```python
from build123d import *

# Parameters (mm, degrees)
F0_W           = 131.6228
F0_H           = 90.3224
F1_DEPTH       = 3
F2_W           = 131.6228
F2_H           = 90.3224
F2_W_2         = 123.6228
F2_H_2         = 82.3224
F3_DEPTH       = 25
F4_W           = 123.6228
F4_H           = 4
F5_DEPTH       = 25
F6_R           = 2.5
F7_W           = 10
F7_H           = 4
F8_DEPTH       = 5
F10_DEPTH      = 25
F10_DEPTH_BACK = 95.8124
F12_D          = 2.5
F12_DEPTH      = 1
F12_TIP        = 0.7510757738
F14_D          = 2.5
F14_DEPTH      = 1
F14_TIP        = 0.7510757738
F16_D          = 2.5
F16_DEPTH      = 1
F16_TIP        = 0.7510757738
F18_D          = 2.5
F18_DEPTH      = 1
F18_TIP        = 0.7510757738
F19_W          = 123.6228
F19_H          = 82.3224
F20_DEPTH      = 3


with BuildPart() as f1:
    # F0 (on Top) → F1 (new body)
    with BuildSketch(Plane.XY):
        Rectangle(F0_W, F0_H)
    extrude(amount=F1_DEPTH)

    # F2 (on face) → F3 (join)
    with BuildSketch(Plane.XY.offset(3)):
        Rectangle(F2_W, F2_H)
        Rectangle(F2_W_2, F2_H_2, mode=Mode.SUBTRACT)
    extrude(amount=F3_DEPTH)

    # F4 (on face) → F5 (join)
    with BuildSketch(Plane.XY.offset(3)):
        Rectangle(F4_W, F4_H)
    extrude(amount=F5_DEPTH)

    # F6
    f6_edges = [f1.edges().sort_by_distance(p)[0] for p in [
        (65.8114, 45.1612, 14),
        (65.8114, -45.1612, 14),
        (-65.8114, -45.1612, 14),
        (-65.8114, 45.1612, 14),
        (0, 45.1612, 0),
        (-65.8114, 0, 0),
        (0, -45.1612, 0),
        (65.8114, 0, 0),
    ]]
    fillet(f6_edges, radius=F6_R)

    # F7 (on face) → F8 (join)
    with BuildSketch(Plane(origin=(0, 45.1612, 0), x_dir=(-1, 0, 0), z_dir=(0, 1, 0))):
        with Locations((-35, 26)):
            Rectangle(F7_W, F7_H)
        with Locations((35, 26)):
            Rectangle(F7_W, F7_H)
    extrude(amount=F8_DEPTH)

    # F9 (on face) → F10 (cut, two sides)
    with BuildSketch(Plane(origin=(30, 0, 0), x_dir=(0, -1, 0), z_dir=(-1, 0, 0))) as f10_sk:
        with BuildLine():
            ThreePointArc((-50.1612, 26), (-49.5754135624, 27.4142135624), (-48.1612, 28))
            Line((-48.1612, 28), (-50.1612, 28))
            Line((-50.1612, 28), (-50.1612, 26))
        make_face()
        with BuildLine():
            Line((-50.1612, 24), (-48.1612, 24))
            ThreePointArc((-48.1612, 24), (-49.5754135624, 24.5857864376), (-50.1612, 26))
            Line((-50.1612, 26), (-50.1612, 24))
        make_face()
        with BuildLine():
            Line((-45.1612, 25), (-46.4291491924, 25))
            ThreePointArc((-46.4291491924, 25), (-47.1612, 24.2679491924), (-48.1612, 24))
            Line((-48.1612, 24), (-45.1612, 24))
            Line((-45.1612, 24), (-45.1612, 25))
        make_face()
        with BuildLine():
            ThreePointArc((-48.1612, 28), (-47.1612, 27.7320508076), (-46.4291491924, 27))
            Line((-46.4291491924, 27), (-45.1612, 27))
            Line((-45.1612, 27), (-45.1612, 28))
            Line((-45.1612, 28), (-48.1612, 28))
        make_face()
    extrude(amount=-F10_DEPTH, mode=Mode.SUBTRACT)
    extrude(f10_sk.sketch, amount=F10_DEPTH_BACK, mode=Mode.SUBTRACT)

    # F12 (one way)
    with BuildSketch(Plane(origin=(30, 0, 0), x_dir=(0, -1, 0), z_dir=(-1, 0, 0))):
        with Locations((-48.1612, 26)):
            Circle(F12_D / 2)
    extrude(amount=-F12_DEPTH, mode=Mode.SUBTRACT)
    with Locations(Plane(origin=(30, 0, 0), x_dir=(0, -1, 0), z_dir=(-1, 0, 0))):
        with Locations((-48.1612, 26)):
            with Locations((0, 0, -(F12_DEPTH + F12_TIP / 2))):  # 118° drill point
                Cone(0, F12_D / 2, F12_TIP, mode=Mode.SUBTRACT)

    # F14
    with Locations(Plane.YZ.offset(40)):
        with Locations((48.1612, 26)):
            Hole(F14_D / 2, depth=F14_DEPTH)
            with Locations((0, 0, -(F14_DEPTH + F14_TIP / 2))):  # 118° drill point
                Cone(0, F14_D / 2, F14_TIP, mode=Mode.SUBTRACT)

    # F16 (one way)
    with BuildSketch(Plane.YZ.offset(-30)):
        with Locations((48.1612, 26)):
            Circle(F16_D / 2)
    extrude(amount=-F16_DEPTH, mode=Mode.SUBTRACT)
    with Locations(Plane.YZ.offset(-30)):
        with Locations((48.1612, 26)):
            with Locations((0, 0, -(F16_DEPTH + F16_TIP / 2))):  # 118° drill point
                Cone(0, F16_D / 2, F16_TIP, mode=Mode.SUBTRACT)

    # F18
    with Locations(Plane(origin=(-40, 0, 0), x_dir=(0, -1, 0), z_dir=(-1, 0, 0))):
        with Locations((-48.1612, 26)):
            Hole(F18_D / 2, depth=F18_DEPTH)
            with Locations((0, 0, -(F18_DEPTH + F18_TIP / 2))):  # 118° drill point
                Cone(0, F18_D / 2, F18_TIP, mode=Mode.SUBTRACT)

    # F19 (on face) → F20 (cut)
    with BuildSketch(Plane.XY.offset(28)):
        Rectangle(F19_W, F19_H)
    extrude(amount=-F20_DEPTH, mode=Mode.SUBTRACT)


solid = f1.part
```
Read the model definition and answer for the solid it produces. Units are mm, in the model's axes. A direction names the side the tool comes from. Coordinates: 2 decimals unless noted, no trailing zeros. Write each loop counter-clockwise with the first axis right and the second up, starting at its lowest first coordinate (ties: lowest second). Pieces come first, ordered by that corner, then holes. Notation, with made-up numbers: (-26, -7.75) -> (19, -7.75) arc R29 ccw to (19, 23.25) -> close; hole circle Ø7 at (58.25, 21.5). An arc over 180 degrees is marked (long way). Return JSON: item names as keys, results as strings.
1. A cutting plane is placed at A-A (y = 10.5). Determine the outline of the cut face in (x, z), and give its area (3 significant figures).
Found:
{"outline": "(-65.81, 2.5) arc R2.5 ccw to (-63.31, 0) -> (63.31, 0) arc R2.5 ccw to (65.81, 2.5) -> (65.81, 28) -> (61.81, 28) -> (61.81, 3) -> (-61.81, 3) -> (-61.81, 28) -> (-65.81, 28) -> close", "area": "592 mm2"}
2. A cutting plane is placed at C-C (x = 58). Determine the outline of the cut face in (y, z).
Found:
{"outline": "(-45.16, 2.5) arc R2.5 ccw to (-42.66, 0) -> (42.66, 0) arc R2.5 ccw to (45.16, 2.5) -> (45.16, 28) -> (41.16, 28) -> (41.16, 3) -> (2, 3) -> (2, 25) -> (-2, 25) -> (-2, 3) -> (-41.16, 3) -> (-41.16, 28) -> (-45.16, 28) -> close"}
3. Find the intervals of material crossed by line 1 along Y through (x, z) = (-31, 8); line 2 along Y through (x, z) = (39.85, 26); line 3 along X through (y, z) = (3, 12), in increasing order. Write a range as from..to.
Found:
{"line 1": "-45.16..-41.16, -2..2, 41.16..45.16", "line 2": "-45.16..-41.16, 41.16..46.91, 49.41..50.16", "line 3": "-65.81..-61.81, 61.81..65.81"}
4. A cutting plane is placed at B-B (z = 8). Determine the outline of the cut face in (x, y).
Found:
{"outline": "(-65.81, -42.66) arc R2.5 ccw to (-63.31, -45.16) -> (63.31, -45.16) arc R2.5 ccw to (65.81, -42.66) -> (65.81, 42.66) arc R2.5 ccw to (63.31, 45.16) -> (-63.31, 45.16) arc R2.5 ccw to (-65.81, 42.66) -> close; hole (-61.81, -41.16) -> (61.81, -41.16) -> (61.81, -2) -> (-61.81, -2) -> close; hole (-61.81, 2) -> (61.81, 2) -> (61.81, 41.16) -> (-61.81, 41.16) -> close"}
5. A tool of negligible diameter and unlimited length cuts with its end or side. For faces 1 (the face through (-39.49, 49.35, 26.38)), 2 (the face through (-30, 47, 27)), 3 (the face through (-1, 22, 3)), 4 (the face through (31.62, 48.38, 26.01)), 5 (the face through (39.49, 49.41, 26.05)), from which of +Z, -Z, +X, -X, +Y, -Y can it reach the whole face along a straight path? Write none if from no direction.
Found:
{"face 1": "-X", "face 2": "+Z, -Z, +Y", "face 3": "+Z", "face 4": "none", "face 5": "+X"}
6. Determine the mould class of faces 6 (the face through (-1, 41.161, 15)), 7 (the face through (38.38, 47.94, 26.01)), 8 (the face through (-1, -2, 14)), 9 (the face through (-1, 1, 0)) for opening direction X: pulls with the +X half, pulls with the -X half, needs draft (parallel to the pull), parting line crosses it, or undercut.
Found:
{"face 6": "undercut", "face 7": "pulls with the +X half", "face 8": "undercut", "face 9": "needs draft"}
7. Each of these flat-tipped pins is pushed along its axis until it touches: P1, Ø6, axis at x = -46, y = 37, coming from the +Z side; P2, Ø7.5, axis at x = 9.5, z = 12, coming from the +Y side; P3, Ø4, axis at y = 48.16, z = 26, coming from the +X side. Where does it stop, or does it pass through?
Found:
{"P1": "z = 3", "P2": "y = 45.16", "P3": "x = 40"}
